Check sheet for the modelled part. Datum: model origin and axes. Units: mm. Face numbers are marked on the shaded views. A direction names the side the tool comes from. Coordinates: 2 decimals unless noted, no trailing zeros. Loops run counter-clockwise (first coordinate to the right, second up) from the corner with the lowest first, then second, coordinate; pieces in that order, holes last. Notation, with made-up numbers: (10, 23.5) - (17, 23.5) arc R26 cw to (17, 49.5) - close; hole circle Ø2 at (71, 17.25). An arc over 180 degrees is marked (long way). Answer as a JSON object with one key per item and string values. Group by question number.
from build123d import *

# Parameters (mm, degrees)
F2_SIZE = 1.5


with BuildPart() as f1:
    # F0 (on Right) → F1 (revolve)
    with BuildSketch(Plane.YZ):
        Polygon((-21, 5.03), (-21, 7.5), (-24, 7.5), (-24, 0), (24, 0), (24, 5.03), (19.1, 5.03), (19.1, 4.8), (18, 4.8), (18, 5.03), align=None)
    revolve(axis=Axis((0, 0, 0), (0, 1, 0)))

    # F2
    f2_edges = [f1.edges().sort_by_distance(p)[0] for p in [
        (0, 24, -5.03),
    ]]
    chamfer(f2_edges, length=F2_SIZE)


solid = f1.part
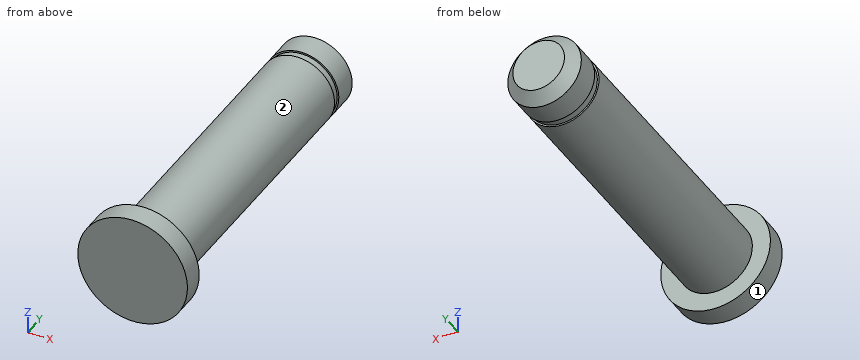
1. Sectioned sample at B-B on z = 0. Record the cut outline in (x, y).
2. Material ranges on line 1 (Y direction, x = -5.5, z = 0.25); line 2 (Y direction, x = 4.5, z = 2); line 3 (Z direction, x = -3.25, y = 8.5), recorded low to high.
3. Sectioned sample at A-A on x = 0. Record the cut outline in (y, z).
4. Gauge pin test, flat ends, axial feed: pin 1 (3 mm diameter, centred on y = 19, z = 6, fed in from -X); pin 2 (4 mm diameter, centred on y = 7.5, z = 0.5, fed in from -X); pin 3 (2 mm diameter, centred on y = -17.5, z = 1, fed in from +X). Record the tip position at first contact, or that the pin passes through.
5. Sectioned sample at C-C on y = -13. Record the cut outline in (x, z).
6. Access from +Z, -Z, +X, -X, +Y, -Y to the whole of each face (thin tool, end or side, straight path). Record for the marked faces 1 and 2.
7. Sectioned sample at D-D on x = -5.75. Record the cut outline in (y, z).
Answers follow:
{
 "1": {"outline": "(-7.5, -24) - (7.5, -24) - (7.5, -21) - (5.03, -21) - (5.03, 18) - (4.8, 18) - (4.8, 19.1) - (5.03, 19.1) - (5.03, 22.5) - (3.53, 24) - (-3.53, 24) - (-5.03, 22.5) - (-5.03, 19.1) - (-4.8, 19.1) - (-4.8, 18) - (-5.03, 18) - (-5.03, -21) - (-7.5, -21) - close"},
 "2": {"line 1": "y = -24 to -21", "line 2": "y = -24 to 18, 19.1 to 22.61", "line 3": "z = -3.84 to 3.84"},
 "3": {"outline": "(-24, -7.5) - (-21, -7.5) - (-21, -5.03) - (18, -5.03) - (18, -4.8) - (19.1, -4.8) - (19.1, -5.03) - (22.5, -5.03) - (24, -3.53) - (24, 3.53) - (22.5, 5.03) - (19.1, 5.03) - (19.1, 4.8) - (18, 4.8) - (18, 5.03) - (-21, 5.03) - (-21, 7.5) - (-24, 7.5) - close"},
 "4": {"pin 1": "stops at x = -2.24", "pin 2": "stops at x = -5.03", "pin 3": "stops at x = 5.03"},
 "5": {"outline": "circle Ø10.06 at (0, 0)"},
 "6": {"face 1": "+Y, -Y", "face 2": "+Y"},
 "7": {"outline": "(-24, -4.82) - (-21, -4.82) - (-21, 4.82) - (-24, 4.82) - close"}
}
